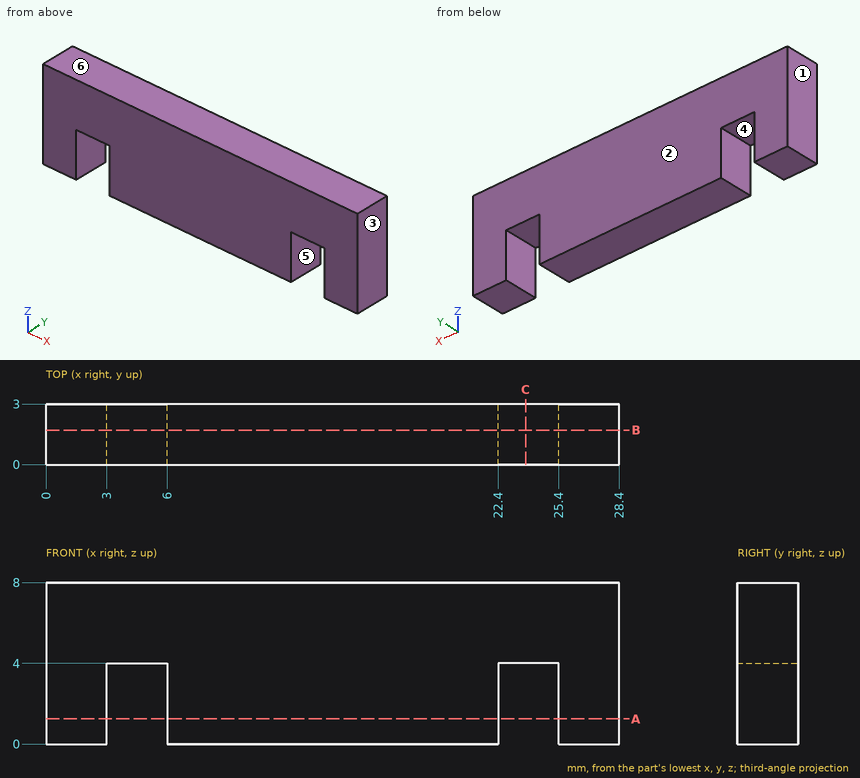
Part print with two shaded views. Sizes in mm from the minimum x, y, z corner. A direction names the side the tool comes from. Round coordinates to 2 decimals unless told otherwise and drop trailing zeros. Loops run counter-clockwise (first coordinate to the right, second up) from the corner with the lowest first, then second, coordinate; pieces in that order, holes last.
Item 1: Saw through at C-C (x = 23.75). List the corners of the cut face in (y, z).
Item 2: Two-plate mould, pull along X, no slides. Class the marked faces 1, 2, 3 and 4: released by +X, released by -X, zero draft, split by the parting line, or undercut.
Item 3: Saw through at A-A (z = 1.25). List the corners of the cut face in (x, y).
Item 4: Which spindle directions (+Z, -Z, +X, -X, +Y, -Y) get a long thin tool onto all of the face, cutting with end or side? Do the marked faces 5 and 6. Say none if no direction does.
Item 5: Saw through at B-B (y = 1.7). List the corners of the cut face in (x, z), then the cut area to 3 significant figures.
Item 6: Drill centre lines: line 1 along X through (y, z) = (1.6, 1); line 2 along Z through (x, y) = (24.75, 0.4). Where is each one in solid material? Low to high.
Worked answers:
1. outline: (0, 4) - (3, 4) - (3, 8) - (0, 8) - close
2. face 1: released by -X
2. face 2: zero draft
2. face 3: released by +X
2. face 4: undercut
3. outline: (0, 0) - (3, 0) - (3, 3) - (0, 3) - close; (6, 0) - (22.4, 0) - (22.4, 3) - (6, 3) - close; (25.4, 0) - (28.4, 0) - (28.4, 3) - (25.4, 3) - close
4. face 5: -Z, +Y, -Y
4. face 6: +Z, +X, -X, +Y, -Y
5. outline: (0, 0) - (3, 0) - (3, 4) - (6, 4) - (6, 0) - (22.4, 0) - (22.4, 4) - (25.4, 4) - (25.4, 0) - (28.4, 0) - (28.4, 8) - (0, 8) - close
5. area: 203 mm2
6. line 1: x = 0 to 3, 6 to 22.4, 25.4 to 28.4
6. line 2: z = 4 to 8
